```python
from build123d import *

# Parameters (mm, degrees)
F0_W     = 50
F0_H     = 50
F2_DEPTH = 2
F3_W     = 20
F3_H     = 20
F4_DEPTH = 25
F5_W     = 2
F5_H     = 16.0369578302
F6_DEPTH = 50
F7_W     = 8.7346149244
F7_H     = 2
F8_DEPTH = 48
F9_DEPTH = 7.3023429058


with BuildPart() as f2:
    # F0 (on Front) → F2 (new body)
    with BuildSketch(Plane.XZ):
        with Locations((25, 25)):
            Rectangle(F0_W, F0_H)
    extrude(amount=F2_DEPTH)

    # F3 (on face) → F4 (cut)
    with BuildSketch(Plane.XZ.offset(2)):
        with Locations((25, 25)):
            Rectangle(F3_W, F3_H)
    extrude(amount=-F4_DEPTH, mode=Mode.SUBTRACT)

    # F5 (on face) → F6 (join, through all)
    with BuildSketch(Plane(origin=(0, 0, 0), x_dir=(1, 0, 0), z_dir=(0, 0, -1))):
        with Locations((49, 10.0184789151)):
            Rectangle(F5_W, F5_H)
    extrude(amount=-F6_DEPTH)

    # F7 (on face) → F8 (join, through all)
    with BuildSketch(Plane(origin=(0, 0, 0), x_dir=(0, -1, 0), z_dir=(-1, 0, 0))):
        with Locations((6.3673074622, 1)):
            Rectangle(F7_W, F7_H)
    extrude(amount=-F8_DEPTH)

    # F9 (add, through all): a face of the model
    f9_faces = [f2.faces().sort_by_distance(p)[0] for p in [
        (24, -10.7346149244, 1),
    ]]
    extrude(f9_faces, amount=F9_DEPTH)


solid = f2.part
```
Part model, mm, in its own coordinate system. A direction names the side the tool comes from. Round coordinates to 2 decimals unless told otherwise and drop trailing zeros. Loops run counter-clockwise (first coordinate to the right, second up) from the corner with the lowest first, then second, coordinate; pieces in that order, holes last. Notation, with made-up numbers: (3, -23) -> (38, -23) arc R17 ccw to (38, -18) -> close; hole circle Ø10 at (-19.75, 75). An arc over 180 degrees is marked (long way). Use one line per item in the form item = value. Start each with the question number.
Item 1: Band-saw the part on B-B (x = 29.5). List the corners of the cut face in (y, z).
Item 2: Band-saw the part on A-A (z = 22). List the corners of the cut face in (x, y).
Item 3: Two-plate mould, pull along Z, no slides. Class faces 1 (the flat face through (25, -1, 35)), 2 (the flat face through (35, -1, 25)), 3 (the flat face through (0, -1.6, 19.3)), 4 (the flat face through (24, -10, 2)): released by +Z, released by -Z, zero draft, split by the parting line, or undercut.
Item 4: Band-saw the part on D-D (y = -16.5). List the corners of the cut face in (x, z).
Item 5: Drill centre lines: line 1 along X through (y, z) = (-5, 33.5); line 2 along Z through (x, y) = (38, -12.25); line 3 along Y through (x, z) = (42, 7). Where is each one in solid material? Low to high.
Item 6: Tool access for faces 5 (the flat face through (48, -10, 26)), 6 (the flat face through (25, -1, 15)), 7 (the flat face through (50, -9, 25)): list every direction of +Z, -Z, +X, -X, +Y, -Y with a clear straight run to the whole face (end or side of a thin tool).
Item 7: Drop flat-ended pins along their axis: pin 1 Ø1.5 at (y, z) = (-6.5, 11) entering from -X; pin 2 Ø5 at (x, z) = (13.5, 34) entering from -Y; pin 3 Ø1.5 at (x, y) = (12.5, -4.5) entering from +Z. Give the stop position or say it passes through.
Item 8: Band-saw the part on C-C (x = 42). List the corners of the cut face in (y, z), plus the area to 3 significant figures.
Data:
q1.outline = (-18.04, 0) -> (0, 0) -> (0, 15) -> (-2, 15) -> (-2, 2) -> (-18.04, 2) -> close; (-2, 35) -> (0, 35) -> (0, 50) -> (-2, 50) -> close
q2.outline = (0, -2) -> (15, -2) -> (15, 0) -> (0, 0) -> close; (35, -2) -> (48, -2) -> (48, -18.04) -> (50, -18.04) -> (50, 0) -> (35, 0) -> close
q3.face_1 = undercut
q3.face_2 = undercut
q3.face_3 = zero draft
q3.face_4 = released by +Z
q4.outline = (0, 0) -> (50, 0) -> (50, 50) -> (48, 50) -> (48, 2) -> (0, 2) -> close
q5.line_1 = 48 to 50
q5.line_2 = 0 to 2
q5.line_3 = -2 to 0
q6.face_5 = +Z, -X, -Y
q6.face_6 = +Y, -Y
q6.face_7 = +Z, -Z, +X, +Y, -Y
q7.pin_1 = 48
q7.pin_2 = -2
q7.pin_3 = 2
q8.outline = (-18.04, 0) -> (0, 0) -> (0, 50) -> (-2, 50) -> (-2, 2) -> (-18.04, 2) -> close
q8.area = 132 mm^2
